```python
from build123d import *

# Parameters (mm, degrees)
BOSS_EXTRU_1_DEPTH             = 3.175
ESQUISSE3_R                    = 2.1
ENL_V_MAT_EXTRU_1_DEPTH        = 48.041658028
ESQUISSE4_W                    = 38.1
ESQUISSE4_H                    = 12.7
ENL_V_MAT_EXTRU_2_DEPTH        = 3.175
CONG_1_R                       = 12.7
CONG_4_R                       = 7.62
CONG_5_R                       = 15.24
BOSS_EXTRU_4_REACH             = 48.719
BOSS_EXTRU_4_DIRECTION_2_REACH = 48.719
CONG_6_R                       = 2.54
BOSS_EXTRU_5_REACH             = 49.042


with BuildPart() as part:
    # Esquisse2 → Boss.-Extru.1 (new, symmetric)
    with BuildSketch(Plane.XY):
        with BuildLine():
            Line((19.05, 0), (28.29484395, 25.4))
            ThreePointArc((28.29484395, 25.4), (22.40844386, 36.409135129), (12.107464983, 29.356433767))
            Line((12.107464983, 29.356433767), (5.08, 11.576433767))
            Line((5.08, 11.576433767), (-5.08, 11.576433767))
            Line((-5.08, 11.576433767), (-12.107464983, 29.356433767))
            ThreePointArc((-12.107464983, 29.356433767), (-22.40844386, 36.409135129), (-28.29484395, 25.4))
            Line((-28.29484395, 25.4), (-19.05, 0))
            Line((-19.05, 0), (-19.05, -12.7))
            Line((-19.05, -12.7), (19.05, -12.7))
            Line((19.05, -12.7), (19.05, 0))
        make_face()
    extrude(amount=BOSS_EXTRU_1_DEPTH, both=True)

    # Esquisse3 → Enlèv. mat.-Extru.1 (cut, through all)
    with BuildSketch(Plane.XY.offset(3.175)):
        with Locations((-20.410216204, 28.244491788)):
            Circle(ESQUISSE3_R)
    enl_v_mat_extru_1 = extrude(amount=-ENL_V_MAT_EXTRU_1_DEPTH, mode=Mode.SUBTRACT)

    # Symétrie1: Enlèv. mat.-Extru.1 across plane
    add(enl_v_mat_extru_1.mirror(Plane(origin=(0, 0, 0), x_dir=(0, 0, 1), z_dir=(1, 0, 0))), mode=Mode.SUBTRACT)

    # Esquisse4 → Enlèv. mat.-Extru.2 (cut)
    with BuildSketch(Plane.XY.offset(3.175)):
        with Locations((0, -6.35)):
            Rectangle(ESQUISSE4_W, ESQUISSE4_H)
    extrude(amount=-ENL_V_MAT_EXTRU_2_DEPTH, mode=Mode.SUBTRACT)

    # Congé1
    # the kernel refuses this fillet: 12.7 mm, written as the material it adds along each edge
    with BuildSketch(Plane(origin=(5.08, 11.576433767, -3.175), x_dir=(0.3675757751944704, 0.9299935749725285, 0), z_dir=(0, 0, 1)), Plane(origin=(-5.08, 11.576433767, -3.175), x_dir=(1, 0, 0), z_dir=(0, 0, 1))) as cong_1_piece_1:
        with BuildLine():
            CenterArc((CONG_1_R * 0.68003074626, CONG_1_R), CONG_1_R, 201.566186537, 68.433813463)
            Line((-CONG_1_R * 0.249962828713, CONG_1_R * 0.632424224806), (0, 0))
            Line((0, 0), (CONG_1_R * 0.68003074626, 0))
        make_face()
    extrude(amount=6.35)

    # Congé4
    cong_4_edges = [part.edges().sort_by_distance(p)[0] for p in [
        (0, 12.084547663, 0),
    ]]
    fillet(cong_4_edges, radius=CONG_4_R)

    # Congé5
    cong_5_edges = [part.edges().sort_by_distance(p)[0] for p in [
        (-19.05, 0, -1.5875),
        (19.05, 0, -1.5875),
    ]]
    fillet(cong_5_edges, radius=CONG_5_R)

    # Boss.-Extru.4: up to this face of the body (flat: up to its plane)
    boss_extru_4_end = Plane(part.part.faces().sort_by_distance((9.3e-08, 10.23403755, -3.175))[0])
    # Esquisse6 → Boss.-Extru.4 (add, up to the picked face)
    with BuildSketch(Plane.XY, mode=Mode.PRIVATE) as boss_extru_4_sk1:
        with BuildLine():
            Line((28.800340403, 28.266812841), (28.800340403, 0))
            Line((28.800340403, 0), (19.288785664, 0))
            ThreePointArc((19.288785664, 0), (19.57466996, 1.27720134), (19.969084459, 2.525163798))
            Line((19.969084459, 2.525163798), (28.29484395, 25.4))
            ThreePointArc((28.29484395, 25.4), (28.672998989, 26.811293816), (28.800340403, 28.266812841))
        make_face()
    boss_extru_4_tool1 = split(extrude(boss_extru_4_sk1.sketch, amount=-BOSS_EXTRU_4_REACH, mode=Mode.PRIVATE), bisect_by=boss_extru_4_end, keep=Keep.BOTH, mode=Mode.PRIVATE)
    boss_extru_4 = boss_extru_4_tool1.solids().sort_by(Axis((25.562927, 8.959806, 0), (0, 0, -1)))[0]
    add(boss_extru_4)

    # Boss.-Extru.4 direction 2: up to this face of the body (flat: up to its plane)
    boss_extru_4_direction_2_end = Plane(part.part.faces().sort_by_distance((7.594682873, 16.877070462, 3.175))[0])
    # Esquisse6 → Boss.-Extru.4 direction 2 (add, up to the picked face)
    with BuildSketch(Plane.XY, mode=Mode.PRIVATE) as boss_extru_4_direction_2_sk1:
        with BuildLine():
            Line((28.800340403, 28.266812841), (28.800340403, 0))
            Line((28.800340403, 0), (19.288785664, 0))
            ThreePointArc((19.288785664, 0), (19.57466996, 1.27720134), (19.969084459, 2.525163798))
            Line((19.969084459, 2.525163798), (28.29484395, 25.4))
            ThreePointArc((28.29484395, 25.4), (28.672998989, 26.811293816), (28.800340403, 28.266812841))
        make_face()
    boss_extru_4_direction_2_tool1 = split(extrude(boss_extru_4_direction_2_sk1.sketch, amount=BOSS_EXTRU_4_DIRECTION_2_REACH, mode=Mode.PRIVATE), bisect_by=boss_extru_4_direction_2_end, keep=Keep.BOTH, mode=Mode.PRIVATE)
    boss_extru_4_direction_2 = boss_extru_4_direction_2_tool1.solids().sort_by(Axis((25.562927, 8.959806, 0), (0, 0, 1)))[0]
    add(boss_extru_4_direction_2)

    # Symétrie3: Boss.-Extru.4, Boss.-Extru.4 direction 2 across plane
    add(boss_extru_4.mirror(Plane(origin=(0, 0, 0), x_dir=(0, 0, 1), z_dir=(1, 0, 0))))
    add(boss_extru_4_direction_2.mirror(Plane(origin=(0, 0, 0), x_dir=(0, 0, 1), z_dir=(1, 0, 0))))

    # Congé6
    cong_6_edges = [part.edges().sort_by_distance(p)[0] for p in [
        (-19.288785664, 0, -1.5875),
        (19.288785664, 0, -1.5875),
    ]]
    fillet(cong_6_edges, radius=CONG_6_R)

    # Esquisse7 → Boss.-Extru.5 (add, up to next)
    with BuildSketch(Plane.XY.offset(3.175), mode=Mode.PRIVATE) as boss_extru_5_sk1:
        with BuildLine():
            Line((-19.288785664, 0), (-19.05, 0))
            Line((-19.05, 0), (-19.969084459, 2.525163798))
            ThreePointArc((-19.969084459, 2.525163798), (-19.57466996, 1.27720134), (-19.288785664, 0))
        make_face()
    boss_extru_5_tool1 = extrude(boss_extru_5_sk1.sketch, amount=-BOSS_EXTRU_5_REACH, mode=Mode.PRIVATE) - part.part
    boss_extru_5 = boss_extru_5_tool1.solids().sort_by_distance((-19.353449, 0.636158, 3.175))[0]
    add(boss_extru_5)

    # Symétrie4: Boss.-Extru.5 across plane
    add(boss_extru_5.mirror(Plane(origin=(0, 0, 0), x_dir=(0, 0, 1), z_dir=(1, 0, 0))))


solid = part.part
```
For this review, take the finished solid that the model builds, in its own axes (mm). A direction names the side the tool comes from. Round coordinates to 2 decimals unless told otherwise and drop trailing zeros. Loops run counter-clockwise (first coordinate to the right, second up) from the corner with the lowest first, then second, coordinate; pieces in that order, holes last.
Q1. Add section D-D on z = 1.25. Give the number of separate pieces and of enclosed holes in the cut face, plus the area to 3 significant figures.
Result sheet:
separate pieces: 1
enclosed holes: 2
area: 1,570 mm2
Q2. Insertion check: pin 1 Ø1 at (y, z) = (-5.5, -1.5) entering from +X; pin 2 Ø6.5 at (x, y) = (7.5, -7) entering from +Z; pin 3 Ø1.5 at (x, z) = (-14, 2) entering from +Y; pin 4 Ø6.5 at (x, y) = (-20.41, 28.24) entering from +Z (3 decimals). Each pin has a flat end and moves straight along its axis. Give the tip position at first contact, or say it passes through.
Result sheet:
pin 1: stops at x = 19.05
pin 2: stops at z = 0
pin 3: stops at y = 34.44
pin 4: stops at z = 3.175
Q3. Machinability: for faces 1 (the face through (20.865, 26.194, 0.044)), 2 (the face through (0, -6, 0)), 3 (the face through (4, 7, -3.175)), 4 (the face through (-19.05, -8, -2)), 5 (the face through (-10.154, 24.414, 0.044)), which of the approach directions +Z, -Z, +X, -X, +Y, -Y give a long, thin tool a straight path to every point of the face, cutting with its end or side? Answer none if there is none.
Result sheet:
face 1: +Z, -Z
face 2: +Z, +X, -X, -Y
face 3: -Z, +X, -X, +Y, -Y
face 4: +Z, -Z, -X, -Y
face 5: +Z, -Z, +Y
Q4. Mouldability with a two-part tool opening along X and no side actions: class faces 6 (the face through (0, 10, 3.175)), 7 (the face through (19.79, -0.75, -1.61)), 8 (the face through (7.005, 17.224, -0.044)) as +X half, -X half, draft (parallel to the pull), parting line (faces both ways), or undercut.
Result sheet:
face 6: draft
face 7: +X half
face 8: undercut
Q5. To check wall thickness, follow line 1 along Z through (x, y) = (12.5, -8.5) (3 decimals); line 2 along X through (y, z) = (25.5, -2.5); line 3 along X through (y, z) = (-10, -2.25). State the ranges of each line that lie inside material, in increasing order.
Result sheet:
line 1: z = -3.175 to 0
line 2: x = -28.8 to -10.58, 10.58 to 28.8
line 3: x = -19.05 to 19.05
Q6. Add section A-A on x = 20.5. Write out the cut boundary in (y, z) (3 decimals).
Result sheet:
outline: (-0.246, -3.175) - (26.146, -3.175) - (26.146, 3.175) - (0, 3.175) - (0, 0) - (-0.246, 0) - close; (30.343, -3.175) - (36.648, -3.175) - (36.648, 3.175) - (30.343, 3.175) - close
Q7. Add section B-B on y = 33. Write out the cut boundary in (x, z) (3 decimals).
Result sheet:
outline: (-27.336, -3.175) - (-13.501, -3.175) - (-13.501, 3.175) - (-27.336, 3.175) - close; (13.501, -3.175) - (27.336, -3.175) - (27.336, 3.175) - (13.501, 3.175) - close
Q8. Add section C-C on x = 9.5. Write out the cut boundary in (y, z) (3 decimals), plus the area to 3 significant figures.
Result sheet:
outline: (-12.7, -3.175) - (22.759, -3.175) - (22.759, 3.175) - (0, 3.175) - (0, 0) - (-12.7, 0) - close
area: 185 mm2
